Work out the finished part from the listing and answer in its coordinate system (mm). A direction names the side the tool comes from. Coordinates: 2 decimals unless noted, no trailing zeros. Order: outer loops, then holes, each group sorted by start corner. A loop starts at its lowest first (then second) coordinate and runs counter-clockwise, first axis right, second up. Notation, with made-up numbers: (0, 55) - (13, 55) arc R18 ccw to (13, 73) - close; hole circle Ø10 at (-19.75, -19.75). An arc over 180 degrees is marked (long way). Use CSV: the item, a comma, the result in double quotes. Start each with the question number.
from build123d import *

# Parameters (mm, degrees)
F0_R      = 5
F1_DEPTH  = 35
F2_W      = 5.05839
F2_H      = 18.62628
F3_DEPTH  = 2.5
F3_FACE_W = 5.05839
F3_FACE_H = 2.5
F4_DEPTH  = 20


with BuildPart() as f1:
    # F0 (on Top) → F1 (new body)
    with BuildSketch(Plane.XY):
        Circle(F0_R)
    extrude(amount=F1_DEPTH)

    # F2 (on face) → F3 (join)
    with BuildSketch(Plane(origin=(0, 0, 0), x_dir=(1, 0, 0), z_dir=(0, 0, -1))):
        with Locations((0, -5)):
            Rectangle(F2_W, F2_H)
    extrude(amount=F3_DEPTH)

    # F3_face (on face) → F4 (join)
    with BuildSketch(Plane(origin=(0, 14.31314, -1.25), x_dir=(-1, 0, 0), z_dir=(0, 1, 0))):
        Rectangle(F3_FACE_W, F3_FACE_H)
    extrude(amount=F4_DEPTH)


solid = f1.part
1) The part is cut by section A-A on y = 0. Determine the outline of the cut face in (x, z), plus the area to 3 significant figures.
2) The part is cut by section D-D on y = 20. Determine the outline of the cut face in (x, z).
3) Flat-ended cylindrical pins translate along their axes: P1, Ø1.5, axis at x = -1, y = 6.5, coming from the +Z side; P2, Ø0.7, axis at x = 4, y = -1.5, coming from the -Z side; P3, Ø1, axis at y = 5, z = 2.5, coming from the -X side; P4, Ø2.5, axis at x = -3.5, y = 1.5, coming from the -Z side. Find the tip coordinate at first contact, or state that the pin passes through.
4) For faces 1 (the face through (-4, 0, 0)), 2 (the face through (0, -4.313, -1)), 3 (the face through (0, 0, 35)), 4 (the face through (0, 34.313, -1)), 5 (the face through (2.529, 15, -1)), determine the directions among +Z, -Z, +X, -X, +Y, -Y from which every point of the face is accessible in a straight line to the end or side of a thin tool.
5) Straight lines are drawn through the part: line 1 (Z direction, x = -0.5, y = 19); line 2 (Y direction, x = 0, z = 10); line 3 (Z direction, x = 2.75, y = -2.5). For each, find the intervals that lie inside material, in ascending order. Write a range as [from, to].
6) The part is cut by section C-C on z = 13.5. Determine the outline of the cut face in (x, y), plus the area to 3 significant figures.
7) The part is cut by section B-B on x = 0. Determine the outline of the cut face in (y, z), plus the area to 3 significant figures.
Answer key:
1,outline,"(-5, 0) - (-2.53, 0) - (-2.53, -2.5) - (2.53, -2.5) - (2.53, 0) - (5, 0) - (5, 35) - (-5, 35) - close"
1,area,"363 mm^2"
2,outline,"(-2.53, -2.5) - (2.53, -2.5) - (2.53, 0) - (-2.53, 0) - close"
3,P1,"z = 0"
3,P2,"z = 0"
3,P3,"x = -2.18"
3,P4,"z = -2.5"
4,face 1,"-Z, -X, +Y, -Y"
4,face 2,"-Z, +X, -X, -Y"
4,face 3,"+Z, +X, -X, +Y, -Y"
4,face 4,"+Z, -Z, +X, -X, +Y"
4,face 5,"-Z, +X, +Y, -Y"
5,line 1,"[-2.5, 0]"
5,line 2,"[-5, 5]"
5,line 3,"[0, 35]"
6,outline,"circle Ø10 at (0, 0)"
6,area,"78.5 mm^2"
7,outline,"(-5, 0) - (-4.31, 0) - (-4.31, -2.5) - (34.31, -2.5) - (34.31, 0) - (5, 0) - (5, 35) - (-5, 35) - close"
7,area,"447 mm^2"
